```python
from build123d import *

# Parameters (mm, degrees)
SKETCH1_W               = 11
SKETCH1_H               = 12
BOSS_EXTRUDE1_DEPTH     = 1.6
SKETCH2_R               = 2
SKETCH2_R_2             = 1
BOSS_EXTRUDE2_DEPTH     = 6
CUT_EXTRUDE1_DEPTH      = 2
CUT_EXTRUDE1_DEPTH_BACK = 2
SKETCH3_R               = 0.5


with BuildPart() as part:
    # Sketch1 → Boss-Extrude1 (new body)
    with BuildSketch(Plane(origin=(0, 0, 0), x_dir=(1, 0, 0), z_dir=(0, 1, 0))):
        Rectangle(SKETCH1_W, SKETCH1_H)
    extrude(amount=BOSS_EXTRUDE1_DEPTH)

    # Sketch2 → Boss-Extrude2 (add)
    # profile 1 of 2: a face of its own
    with BuildSketch(Plane(origin=(0, 1.6, 0), x_dir=(1, 0, 0), z_dir=(0, 1, 0))):
        with Locations(Location((-3, 0, 0), (0, 0, 270))):
            Circle(SKETCH2_R)
        with Locations(Location((-3, 0, 0), (0, 0, 270))):
            Circle(SKETCH2_R_2, mode=Mode.SUBTRACT)
    # profile 2 of 2: a face of its own
    with BuildSketch(Plane(origin=(0, 1.6, 0), x_dir=(1, 0, 0), z_dir=(0, 1, 0))):
        with Locations(Location((3, 0, 0), (0, 0, 270))):
            Circle(SKETCH2_R)
        with Locations(Location((3, 0, 0), (0, 0, 270))):
            Circle(SKETCH2_R_2, mode=Mode.SUBTRACT)
    extrude(amount=BOSS_EXTRUDE2_DEPTH)

    # Sketch3 → Cut-Extrude1 (cut, two sides: drawn at the far end of the back side and taken through both)
    with BuildSketch(Plane.XY.offset(-CUT_EXTRUDE1_DEPTH_BACK)):
        with Locations(Location((-3, 6.6, 0), (0, 0, 270.000000002))):
            Circle(SKETCH3_R)
        with Locations(Location((3, 6.6, 0), (0, 0, 270.000000002))):
            Circle(SKETCH3_R)
    extrude(amount=CUT_EXTRUDE1_DEPTH + CUT_EXTRUDE1_DEPTH_BACK, mode=Mode.SUBTRACT)


solid = part.part
```
Source: CAD feature listing. Evaluate the final solid. Frame: model axes, mm. A direction names the side the tool comes from. Coordinates: 2 decimals unless noted, no trailing zeros. Loops run counter-clockwise (first coordinate to the right, second up) from the corner with the lowest first, then second, coordinate; pieces in that order, holes last. Notation, with made-up numbers: M -31,8.5 L 25,8.5 A25 cw 25,36.5 Z; hole C 21,32.25 d9. An arc over 180 degrees is marked long. Use a Markdown table: item, result. Add a question column.
Q1. Draft query along Z for faces 3 (the cylindrical face through (-3.766, 4.558, 1.847)), 4 (the flat face through (5.5, 1, 0)), 5 (the cylindrical face through (3, 5, -1)). Return one class per face: pulls with the +Z half, pulls with the -Z half, needs draft (parallel to the pull), parting line crosses it, or undercut.
Q2. Section query C-C, the plane z = 0. Return loops of the section in (x, y), and give its area (3 significant figures).
Q3. Access query for faces 1 (the flat face through (3, 1.6, 0)), 2 (the cylindrical face through (-2.85, 6.123, -1.441)). Directions: +Z, -Z, +X, -X, +Y, -Y. A direction counts if a zero-diameter tool reaches every point of the face in a straight line with its end or side. Return the directions, or none.
Q4. Section query D-D, the plane y = 6.6. Return loops of the section in (x, z).
Q5. Section query B-B, the plane y = 5.5. Return loops of the section in (x, z), and give its area (3 significant figures).
Q6. Material intervals for L1, parallel to X at y = 4.75, z = 0; L2, parallel to X at y = 6.6, z = 1.25; L3, parallel to Z at x = 2.25, y = 1.75, sorted ascending.
Q7. Section query A-A, the plane x = -3. Return loops of the section in (y, z).
Result:
| question | item | result |
|---|---|---|
| 1 | face 3 | parting line crosses it |
| 1 | face 4 | needs draft |
| 1 | face 5 | undercut |
| 2 | outline | M -5.5,0 L 5.5,0 L 5.5,1.6 L 5,1.6 L 5,7.6 L 4,7.6 L 4,1.6 L 2,1.6 L 2,7.6 L 1,7.6 L 1,1.6 L -1,1.6 L -1,7.6 L -2,7.6 L -2,1.6 L -4,1.6 L -4,7.6 L -5,7.6 L -5,1.6 L -5.5,1.6 Z |
| 2 | area | 41.6 mm2 |
| 3 | face 1 | +Y |
| 3 | face 2 | +Z, -Z |
| 4 | outline | M -3.5,-1.94 L -3.5,-0.87 A1 cw -3.5,0.87 L -3.5,1.94 A2 ccw Z; M -2.5,-1.94 A2 ccw -2.5,1.94 L -2.5,0.87 A1 cw -2.5,-0.87 Z; M 2.5,-1.94 L 2.5,-0.87 A1 cw 2.5,0.87 L 2.5,1.94 A2 ccw Z; M 3.5,-1.94 A2 ccw 3.5,1.94 L 3.5,0.87 A1 cw 3.5,-0.87 Z |
| 5 | outline | C -3,0 d4; C 3,0 d4; hole C -3,0 d2; hole C 3,0 d2 |
| 5 | area | 18.8 mm2 |
| 6 | L1 | x = -5 to -4, -2 to -1, 1 to 2, 4 to 5 |
| 6 | L2 | x = -4.56 to -3.5, -2.5 to -1.44, 1.44 to 2.5, 3.5 to 4.56 |
| 6 | L3 | z = -1.85 to -0.66, 0.66 to 1.85 |
| 7 | outline | M 0,-6 L 1.6,-6 L 1.6,-2 L 6.1,-2 L 6.1,-1 L 1.6,-1 L 1.6,1 L 6.1,1 L 6.1,2 L 1.6,2 L 1.6,6 L 0,6 Z; M 7.1,-2 L 7.6,-2 L 7.6,-1 L 7.1,-1 Z; M 7.1,1 L 7.6,1 L 7.6,2 L 7.1,2 Z |
